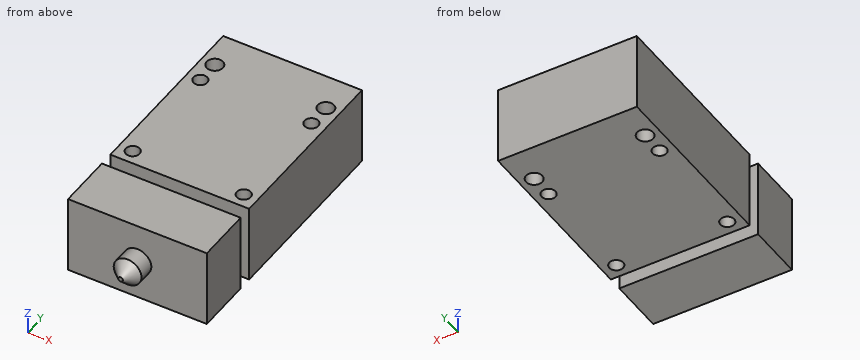
Autodesk Inventor part; units mm, degrees
ref_plane "YZ Plane" through (0, 0, 0) normal (1, 0, 0) x (0, 1, 0)
ref_plane "XZ Plane" through (0, 0, 0) normal (0, 1, 0) x (-1, 0, 0)
ref_plane "XY Plane" through (0, 0, 0) normal (0, 0, 1) x (1, 0, 0)
sketch "Boceto1" plane through (0, 0, 0) normal (0, 0, 1) x (1, 0, 0)
  line L0 (-15, 20) -> (15, 20)
  line L1 (15, 20) -> (15, -20)
  line L2 (15, -20) -> (-15, -20)
  line L3 (-15, -20) -> (-15, 20)
  line L4 (5.2741, 0) -> (0, 0)
  line L5 (0, 0) -> (0, 2.4047)
  dimension "d0" = 30
  dimension "d1" = 40
extrude "Extrusión1" add sketch "Boceto1" along normal blind 17
sketch "Boceto2" plane through (0, 0, 17) normal (0, 0, 1) x (1, 0, 0)
  circle A0 centre (12, -17) radius 1.5
  line L0 (15, -20) -> (15, 20)
  line L1 (-15, -20) -> (15, -20)
  circle A1 centre (12, 7) radius 1.5
  circle A2 centre (12, 12.1331) radius 1.75
  point P0 (0, 0)
  dimension "d4" = 3
  dimension "d5" = 3
  dimension "d6" = 3
  dimension "d7" = 3
  dimension "d8" = 3
  dimension "d9" = 24
  dimension "d10" = 3.5
  dimension "d11" = 3
extrude "Extrusión2" cut sketch "Boceto2" against normal through all
mirror "Simetría1" about plane through (0, 0, 0) normal (1, 0, 0) of "Extrusión2"
sketch "Boceto3" plane through (0, 0, 17) normal (0, 0, 1) x (1, 0, 0)
  line L0 (-15, -23) -> (15, -23)
  line L1 (15, -23) -> (15, -35)
  line L2 (15, -35) -> (-15, -35)
  line L3 (-15, -35) -> (-15, -23)
  line L4 (-15, -20) -> (15, -20)
  point P0 (0, 0)
  dimension "d14" = 12
  dimension "d22" = 3
extrude "Extrusión3" add sketch "Boceto3" against normal up to surface (17 mm away)
sketch "Boceto4" plane through (0, 0, 0) normal (1, 0, 0) x (0, 1, 0)
  line L0 (-38.5, 5.5) -> (-35, 5.5)
  line L1 (-35, 17) -> (-35, 0)
  line L2 (-23, 0) -> (-35, 0)
  line L3 (-23, 17) -> (-23, 0)
  line L4 (-23, 5.5) -> (-20, 5.5)
  line L5 (-20, 0) -> (-20, 17)
  line L6 (-41, 8.5) -> (-20, 8.5)
  line L7 (-41, 8.5) -> (-41, 8)
  line L8 (-41, 8) -> (-38.5, 5.5)
  point P0 (0, 0)
  point P1 (-35, 8.5)
  point P2 (-23, 8.5)
  dimension "d18" = 6
  dimension "d19" = 3
  dimension "d20" = 8.5
  dimension "d23" = 0.5
  dimension "d24" = 135
revolve "Revolución1" add sketch "Boceto4" angle 360 about axis through (0, -41, 8.5) along (0, 1, 0) contours L8 L7 L6 L1 L0 | L6 L5 L4 L3
equation "\"d7\" = d4"
equation "\"d8\" = d5"
equation "\"d11\" = d8"
properties part number "NF TC-02" material "Cobre, aleado"
Here's how the part is built. I have some questions about the finished solid (model axes, mm). Coordinates: 2 decimals unless noted, no trailing zeros. Loops run counter-clockwise (first coordinate to the right, second up) from the corner with the lowest first, then second, coordinate; pieces in that order, holes last. Notation, with made-up numbers: M 41,38.5 L 75,38.5 A7 ccw 75,43.5 Z; hole C 85,77.5 d5. An arc over 180 degrees is marked long. One line per item, written item: value.
1. Imagine slicing it at D-D (x = 4.5). List the corners of the cut face in (y, z) for me.
Geometry says:
outline: M -35,0 L -23,0 L -23,17 L -35,17 Z; M -20,0 L 20,0 L 20,17 L -20,17 Z
2. Will these pins go through, and if not, where does the flat tip stop? pin 1 Ø8.5 at (x, z) = (6, 6.5) entering from -Y; pin 2 Ø2.5 at (x, y) = (12, 7) entering from +Z; pin 3 Ø8 at (x, z) = (-8, 8.5) entering from -Y.
Geometry says:
pin 1: stops at y = -39.43
pin 2: passes through
pin 3: stops at y = -35
3. Imagine slicing it at C-C (x = 12). List the corners of the cut face in (y, z) for me, and give its area (4 significant figures).
Geometry says:
outline: M -35,0 L -23,0 L -23,17 L -35,17 Z; M -20,0 L -18.5,0 L -18.5,17 L -20,17 Z; M -15.5,0 L 5.5,0 L 5.5,17 L -15.5,17 Z; M 8.5,0 L 10.38,0 L 10.38,17 L 8.5,17 Z; M 13.88,0 L 20,0 L 20,17 L 13.88,17 Z
area: 722.5 mm2
4. Imagine slicing it at B-B (z = 3). List the corners of the cut face in (x, y) for me.
Geometry says:
outline: M -15,-35 L 15,-35 L 15,-23 L -15,-23 Z; M -15,-20 L 15,-20 L 15,20 L -15,20 Z; hole C -12,12.13 d3.5; hole C -12,-17 d3; hole C -12,7 d3; hole C 12,12.13 d3.5; hole C 12,-17 d3; hole C 12,7 d3
5. Please list where these lines run through material, in increasing order: probe 1 along Y at (x, z) = (12, 12.75); probe 2 along Y at (x, z) = (-11, 2.75); probe 3 along Y at (x, z) = (-4, 8.75).
Geometry says:
probe 1: y = -35 to -23, -20 to -18.5, -15.5 to 5.5, 8.5 to 10.38, 13.88 to 20
probe 2: y = -35 to -23, -20 to -18.12, -15.88 to 5.88, 8.12 to 10.7, 13.57 to 20
probe 3: y = -35 to -23, -20 to 20
6. Imagine slicing it at A-A (y = -17). List the corners of the cut face in (x, z) for me, and give its area (3 significant figures).
Geometry says:
outline: M -15,0 L -13.5,0 L -13.5,17 L -15,17 Z; M -10.5,0 L 10.5,0 L 10.5,17 L -10.5,17 Z; M 13.5,0 L 15,0 L 15,17 L 13.5,17 Z
area: 408 mm2
